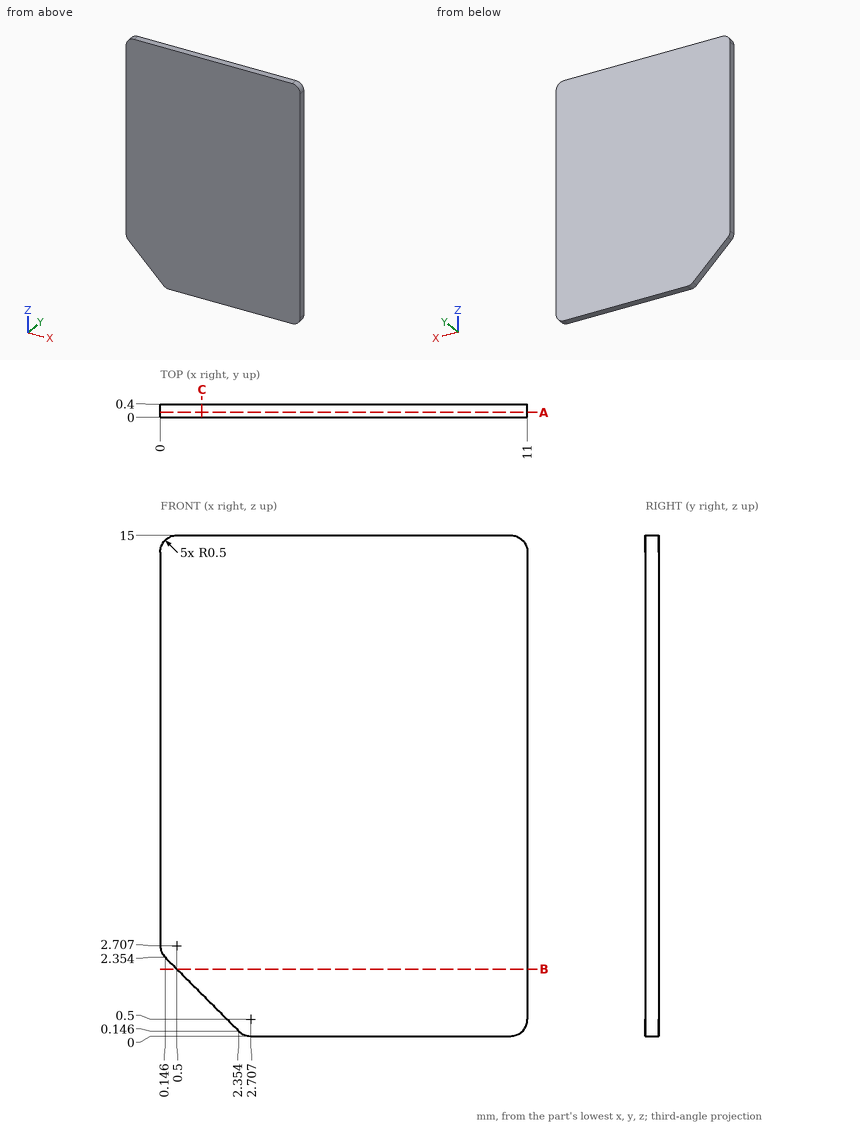
Print and shaded views of the part. All mm, measured from the part's lowest x, y and z. Round coordinates to 2 decimals unless told otherwise and drop trailing zeros. Write each loop counter-clockwise with the first axis right and the second up, starting at its lowest first coordinate (ties: lowest second). Pieces come first, ordered by that corner, then holes. Notation, with made-up numbers: (87.25, -27.75) -> (93.25, -27.75) arc R20 ccw to (93.25, 1.25) -> close; hole circle Ø2 at (66, 76.5). An arc over 180 degrees is marked (long way). Answer in a Markdown table with one row per item. Add a question column.
Item 1: Saw through at B-B, the plane z = 2. Write the cut outline in (x, y).
Item 2: Saw through at C-C, the plane x = 1.25. Write the cut outline in (y, z).
Item 3: Drill centre lines: line 1 (X direction, y = 0.2, z = 2); line 2 (X direction, y = 0.3, z = 0.75). Where is each one in solid material? Low to high. Write a range as from..to.
Item 4: Saw through at A-A, the plane y = 0.15. Write the cut outline in (x, z), then the cut area to 3 significant figures.
Findings below:
| question | item | result |
|---|---|---|
| 1 | outline | (0.5, 0) -> (11, 0) -> (11, 0.4) -> (0.5, 0.4) -> close |
| 2 | outline | (0, 1.25) -> (0.4, 1.25) -> (0.4, 15) -> (0, 15) -> close |
| 3 | line 1 | x = 0.5..11 |
| 3 | line 2 | x = 1.75..11 |
| 4 | outline | (0, 2.71) arc R0.5 ccw to (0.15, 2.35) -> (2.35, 0.15) arc R0.5 ccw to (2.71, 0) -> (10.5, 0) arc R0.5 ccw to (11, 0.5) -> (11, 14.5) arc R0.5 ccw to (10.5, 15) -> (0.5, 15) arc R0.5 ccw to (0, 14.5) -> close |
| 4 | area | 162 mm^2 |
